from build123d import *

# Parameters (mm, degrees)
FILLET_1_R = 0.2


with BuildPart() as part:
    # 草图1 → 旋转-薄壁1 (revolve)
    with BuildSketch(Plane.XY):
        Polygon((3.5, -11.099526066), (7.5, -11.099526066), (7.5, 5.900473934), (0, 5.900473934), (0, 5.300473934), (6.9, 5.300473934), (6.9, -10.499526066), (3.5, -10.499526066), align=None)
    revolve(axis=Axis((0, -19.840377492, 0), (0, 1, 0)))

    # 草图3 → M2 螺纹孔1 (revolve, cut)
    with BuildSketch(Plane(origin=(0, -11.099526066, -5.439713429), x_dir=(0, 0, -1), z_dir=(1, 0, 0))):
        Polygon((0, 0), (0, 2.480688495), (0.8, 2), (0.8, 0), align=None)
    hole_wizard_m2_1 = revolve(axis=Axis((0, -17.449526066, -5.439713429), (0, 1, 0)), mode=Mode.SUBTRACT)

    # 镜向1: M2 螺纹孔1 across plane
    add(hole_wizard_m2_1.mirror(Plane.XY), mode=Mode.SUBTRACT)

    # 圆角1
    fillet_1_edges = [part.edges().sort_by_distance(p)[0] for p in [
        (-7.5, -11.099526066, 0),
    ]]
    fillet(fillet_1_edges, radius=FILLET_1_R)


solid = part.part
For this review, take the finished solid that the model builds, in its own axes (mm). A direction names the side the tool comes from. Round coordinates to 2 decimals unless told otherwise and drop trailing zeros. Loops run counter-clockwise (first coordinate to the right, second up) from the corner with the lowest first, then second, coordinate; pieces in that order, holes last. Notation, with made-up numbers: (13.5, 7.25) - (54.5, 7.25) arc R22 ccw to (54.5, 32.25) - close; hole circle Ø7 at (22.5, 65). An arc over 180 degrees is marked (long way). Answer as CSV lines item,"result".
(1) Consider section C-C on y = -1.5. Give the boundary of the cut face in (x, z).
Checked values:
outline,"circle Ø15 at (0, 0); hole circle Ø13.8 at (0, 0)"
(2) Consider section B-B on z = 0. Give the boundary of the cut face in (x, y).
Checked values:
outline,"(-7.5, -10.9) arc R0.2 ccw to (-7.3, -11.1) - (-3.5, -11.1) - (-3.5, -10.5) - (-6.9, -10.5) - (-6.9, 5.3) - (6.9, 5.3) - (6.9, -10.5) - (3.5, -10.5) - (3.5, -11.1) - (7.3, -11.1) arc R0.2 ccw to (7.5, -10.9) - (7.5, 5.9) - (-7.5, 5.9) - close"
(3) Wall thickness on line 1 (Z direction, x = 0, y = -10.8); line 2 (Y direction, x = 4.5, z = 3.5); line 3 (X direction, y = -10.8, z = 0): over which ranges is each line inside the solid? List them lowest first.
Checked values:
line 1,"z = -7.5 to -6.24, -4.64 to -3.5, 3.5 to 4.64, 6.24 to 7.5"
line 2,"y = -11.1 to -10.5, 5.3 to 5.9"
line 3,"x = -7.5 to -3.5, 3.5 to 7.5"
(4) Consider section A-A on x = 0. Give the boundary of the cut face in (y, z).
Checked values:
outline,"(-11.1, -7.3) arc R0.2 ccw to (-10.9, -7.5) - (5.9, -7.5) - (5.9, 7.5) - (-10.9, 7.5) arc R0.2 ccw to (-11.1, 7.3) - (-11.1, 6.24) - (-10.5, 6.24) - (-10.5, 6.9) - (5.3, 6.9) - (5.3, -6.9) - (-10.5, -6.9) - (-10.5, -6.24) - (-11.1, -6.24) - close; (-11.1, -4.64) - (-10.5, -4.64) - (-10.5, -3.5) - (-11.1, -3.5) - close; (-11.1, 3.5) - (-10.5, 3.5) - (-10.5, 4.64) - (-11.1, 4.64) - close"
(5) Tool access review of faces 4 (the face through (-7.493, -2.382, -0.33)), 5 (the face through (-0.04, -10.8, -4.64)), 6 (the face through (-0.9, -2.71, -6.84)): name each direction out of +Z, -Z, +X, -X, +Y, -Y from which nothing blocks a thin tool from reaching the whole face with its end or side.
Checked values:
face 4,"+Y, -Y"
face 5,"-Y"
face 6,"none"
(6) Insertion check: P1, Ø8, axis at x = -4.5, y = 3.5, coming from the +Z side; P2, Ø1.4, axis at x = 0, z = 5.44, coming from the -Y side; P3, Ø2, axis at y = 1.5, z = -4.5, coming from the +X side. Each pin has a flat end and moves straight along its axis. Give the tip position at first contact, or say it passes through.
Checked values:
P1,"stops at z = 7.48"
P2,"stops at y = 5.3"
P3,"stops at x = 6.63"
(7) Mouldability with a two-part tool opening along Y and no side actions: class faces 1 (the face through (3, -10.5, 3)), 2 (the face through (3.35, -11.1, 1.52)), 3 (the face through (-0.04, -10.8, 4.64)) as +Y half, -Y half, draft (parallel to the pull), parting line (faces both ways), or undercut.
Checked values:
face 1,"undercut"
face 2,"-Y half"
face 3,"draft"
